Check sheet for the modelled part. Datum: model origin and axes. Units: mm. A direction names the side the tool comes from. Coordinates: 2 decimals unless noted, no trailing zeros. Write each loop counter-clockwise with the first axis right and the second up, starting at its lowest first coordinate (ties: lowest second). Pieces come first, ordered by that corner, then holes. Notation, with made-up numbers: (-28.75, 58.5) - (-23.75, 58.5) arc R19 ccw to (-23.75, 80.5) - close; hole circle Ø8 at (86, -31.75). An arc over 180 degrees is marked (long way). Write each question's results on one line, items separated by ' | '.
from build123d import *

# Parameters (mm, degrees)
EXTRUDE_1_DEPTH     = 50
CUT_EXTRUDE_2_DEPTH = 30
CHAMFER_1_SIZE      = 2


with BuildPart() as part:
    # 草图1 → 凸台-拉伸1 (new body)
    with BuildSketch(Plane(origin=(0, 0, 0), x_dir=(1, 0, 0), z_dir=(0, 1, 0))):
        with BuildLine():
            Line((-158, -160), (158, -160))
            ThreePointArc((158, -160), (159.414213562, -159.414213562), (160, -158))
            Line((160, -158), (160, 158))
            ThreePointArc((160, 158), (159.414213562, 159.414213562), (158, 160))
            Line((158, 160), (-158, 160))
            ThreePointArc((-158, 160), (-159.414213562, 159.414213562), (-160, 158))
            Line((-160, 158), (-160, -158))
            ThreePointArc((-160, -158), (-159.414213562, -159.414213562), (-158, -160))
        make_face()
    extrude(amount=-EXTRUDE_1_DEPTH)

    # 草图2 → 切除-拉伸2 (cut)
    with BuildSketch(Plane(origin=(0, 0, 0), x_dir=(1, 0, 0), z_dir=(0, 1, 0))):
        with BuildLine():
            Line((130, -153), (130, -160))
            Line((130, -160), (-130, -160))
            Line((-130, -160), (-130, -153))
            ThreePointArc((-130, -153), (-129.121320344, -150.878679656), (-127, -150))
            Line((-127, -150), (-110, -150))
            ThreePointArc((-110, -150), (-102.928932188, -147.071067812), (-100, -140))
            Line((-100, -140), (-100, 80))
            ThreePointArc((-100, 80), (-97.071067812, 87.071067812), (-90, 90))
            Line((-90, 90), (90, 90))
            ThreePointArc((90, 90), (97.071067812, 87.071067812), (100, 80))
            Line((100, 80), (100, -140))
            ThreePointArc((100, -140), (102.928932188, -147.071067812), (110, -150))
            Line((110, -150), (127, -150))
            ThreePointArc((127, -150), (129.121320344, -150.878679656), (130, -153))
        make_face()
    extrude(amount=-CUT_EXTRUDE_2_DEPTH, mode=Mode.SUBTRACT)

    # 倒角1
    chamfer_1_edges = [part.edges().sort_by_distance(p)[0] for p in [
        (130, 0, 156.5),
        (129.121320344, 0, 150.878679656),
        (118.5, 0, 150),
        (102.928932188, 0, 147.071067812),
        (100, 0, 30),
        (97.071067812, 0, -87.071067812),
        (0, 0, -90),
        (-97.071067812, 0, -87.071067812),
        (-100, 0, 30),
        (-102.928932188, 0, 147.071067812),
        (-118.5, 0, 150),
        (-129.121320344, 0, 150.878679656),
        (-130, 0, 156.5),
    ]]
    chamfer(chamfer_1_edges, length=CHAMFER_1_SIZE)


solid = part.part
1. Go/stop test with flat-tipped pins: pin 1 (12 mm diameter, centred on x = -33.5, y = -6, fed in from +Z); pin 2 (3 mm diameter, centred on x = 7, z = -40.5, fed in from +Y); pin 3 (18.5 mm diameter, centred on x = -117.5, y = -15, fed in from +Z). Record where each tip stops, or that it passes through.
Values follow:
pin 1: stops at z = -90 | pin 2: stops at y = -30 | pin 3: stops at z = 150
2. Access from +Z, -Z, +X, -X, +Y, -Y to the whole of each face (thin tool, end or side, straight path). Record for faces 1 (the cylindrical face through (-97.15, -15.8, -86.99)), 2 (the flat face through (160, -25, 2)).
Values follow:
face 1: +Z, +Y | face 2: +Z, -Z, +X, +Y, -Y
3. Sectioned sample at B-B (x = 116). Record the cut outline in (y, z), then the cut area to 3 significant figures.
Values follow:
outline: (-50, -160) - (0, -160) - (0, 148) - (-2, 150) - (-30, 150) - (-30, 160) - (-50, 160) - close | area: 15,700 mm^2
4. Material ranges on L1, parallel to X at y = -19, z = -74; L2, parallel to Y at x = 10, z = -75.5; L3, parallel to Z at x = -126, y = -10, recorded low to high. Write a range as [from, to].
Values follow:
L1: x = [-160, -100], [100, 160] | L2: y = [-50, -30] | L3: z = [-160, 150]
5. Sectioned sample at A-A (z = 87.5). Record the cut outline in (x, y), then the cut area to 4 significant figures.
Values follow:
outline: (-160, -50) - (160, -50) - (160, 0) - (102, 0) - (100, -2) - (100, -30) - (-100, -30) - (-100, -2) - (-102, 0) - (-160, 0) - close | area: 10,000 mm^2
6. Sectioned sample at C-C (y = -21). Record the cut outline in (x, z).
Values follow:
outline: (-160, -158) arc R2 ccw to (-158, -160) - (158, -160) arc R2 ccw to (160, -158) - (160, 158) arc R2 ccw to (158, 160) - (130, 160) - (130, 153) arc R3 cw to (127, 150) - (110, 150) arc R10 ccw to (100, 140) - (100, -80) arc R10 cw to (90, -90) - (-90, -90) arc R10 cw to (-100, -80) - (-100, 140) arc R10 ccw to (-110, 150) - (-127, 150) arc R3 cw to (-130, 153) - (-130, 160) - (-158, 160) arc R2 ccw to (-160, 158) - close
7. Sectioned sample at D-D (x = 34.5). Record the cut outline in (y, z).
Values follow:
outline: (-50, -160) - (0, -160) - (0, -92) - (-2, -90) - (-30, -90) - (-30, 160) - (-50, 160) - close
8. Draft check along X on faces 3 (the flat face through (130, -16, 156)), 4 (the flat face through (-2, -36, 160)), 5 (the flat face through (-119, -16, 150)), 6 (the flat face through (-160, -25, -2)). Enter one of: pulls with the +X half, pulls with the -X half, needs draft (parallel to the pull), parting line crosses it, or undercut.
Values follow:
face 3: undercut | face 4: needs draft | face 5: undercut | face 6: pulls with the -X half
